from build123d import *

# Parameters (mm, degrees)
EXTRUDE_1_DEPTH        = 20
EXTRUDE_2_DEPTH        = 70
F_1_4_BASE_D           = 3.4
F_1_4_BASE_CBORE_D     = 6.7
F_1_4_BASE_CBORE_DEPTH = 1.65
SKETCH_11_W            = 22
SKETCH_11_H            = 42
CUT_EXTRUDE_1_DEPTH    = 32
CUT_EXTRUDE_2_DEPTH    = 67
SKETCH_15_R            = 5
CUT_EXTRUDE_3_DEPTH    = 70
CUT_EXTRUDE_4_DEPTH    = 2
CUT_EXTRUDE_5_DEPTH    = 3.5


with BuildPart() as part:
    # 草图1 → 凸台-拉伸1 (new body)
    with BuildSketch(Plane(origin=(0, 0, 0), x_dir=(1, 0, 0), z_dir=(0, 1, 0))):
        with BuildLine():
            Line((75.055476805, 35), (35.707142143, 35))
            ThreePointArc((35.707142143, 35), (46.289075964, 18.902948088), (50, 0))
            ThreePointArc((50, 0), (46.289075964, -18.902948088), (35.707142143, -35))
            Line((35.707142143, -35), (75.055476805, -35))
            Line((75.055476805, -35), (75.055476805, 35))
        make_face()
        with BuildLine():
            Line((0.055476805, -35), (0.055476805, 35))
            Line((0.055476805, 35), (35.707142143, 35))
            ThreePointArc((35.707142143, 35), (-50, 0), (35.707142143, -35))
            Line((35.707142143, -35), (0.055476805, -35))
        make_face()
        with BuildLine():
            Line((35.707142143, 35), (0.055476805, 35))
            Line((0.055476805, 35), (0.055476805, -35))
            Line((0.055476805, -35), (35.707142143, -35))
            ThreePointArc((35.707142143, -35), (46.289075964, -18.902948088), (50, 0))
            ThreePointArc((50, 0), (46.289075964, 18.902948088), (35.707142143, 35))
        make_face()
    extrude_1 = extrude(amount=EXTRUDE_1_DEPTH)

    # 草图2 → 凸台-拉伸2 (add)
    with BuildSketch(Plane.XY.offset(35)):
        Polygon((75.055476805, 0), (140.174133177, 114.192122372), (140.174133177, 191.411564081), (120.174133177, 191.411564081), (120.174133177, 109.286292207), (75.055476805, 20), align=None)
    extrude_2 = extrude(amount=-EXTRUDE_2_DEPTH)

    # 镜向1: 凸台-拉伸1, 凸台-拉伸2 across plane
    add(extrude_1.mirror(Plane(origin=(0, 0, 0), x_dir=(0, 0, 1), z_dir=(1, 0, 0))))
    add(extrude_2.mirror(Plane(origin=(0, 0, 0), x_dir=(0, 0, 1), z_dir=(1, 0, 0))))

    # 1/4 六角头螺钉的柱形沉头孔base (through all)
    with Locations(Plane(origin=(0, 20, 0), x_dir=(1, 0, 0), z_dir=(0, 1, 0))):
        with Locations((0, 0)):
            CounterBoreHole(F_1_4_BASE_D / 2, F_1_4_BASE_CBORE_D / 2, F_1_4_BASE_CBORE_DEPTH)

    # 草图11 → 切除-拉伸1 (cut)
    with BuildSketch(Plane(origin=(140.174133177, 0, 0), x_dir=(0, 0, -1), z_dir=(1, 0, 0))):
        with Locations((0, 152.801564081)):
            Rectangle(SKETCH_11_W, SKETCH_11_H)
    extrude(amount=-CUT_EXTRUDE_1_DEPTH, mode=Mode.SUBTRACT)

    # 草图14 → 切除-拉伸2 (cut)
    with BuildSketch(Plane(origin=(140.174133177, 0, 0), x_dir=(0, 0, -1), z_dir=(1, 0, 0))):
        with BuildLine():
            Line((-10, 179.101564081), (10, 179.101564081))
            ThreePointArc((10, 179.101564081), (11, 178.101564081), (10, 177.101564081))
            Line((10, 177.101564081), (-10, 177.101564081))
            ThreePointArc((-10, 177.101564081), (-11, 178.101564081), (-10, 179.101564081))
        make_face()
        with BuildLine():
            Line((-10, 128.501564081), (8.706275956, 128.501564081))
            ThreePointArc((8.706275956, 128.501564081), (9.706275956, 127.501564081), (8.706275956, 126.501564081))
            Line((8.706275956, 126.501564081), (-10, 126.501564081))
            ThreePointArc((-10, 126.501564081), (-11, 127.501564081), (-10, 128.501564081))
        make_face()
    extrude(amount=-CUT_EXTRUDE_2_DEPTH, mode=Mode.SUBTRACT)

    # 草图15 → 切除-拉伸3 (cut)
    with BuildSketch(Plane.ZY.offset(140.174133177)):
        with Locations((0, 172.801564081)):
            Circle(SKETCH_15_R)
    extrude(amount=-CUT_EXTRUDE_3_DEPTH, mode=Mode.SUBTRACT)

    # 草图16 → 切除-拉伸4 (cut)
    with BuildSketch(Plane.XZ):
        with BuildLine():
            Line((-30, 3), (0.784894819, 6.64557965))
            Line((0.784894819, 6.64557965), (31.544487342, 2.792338441))
            ThreePointArc((31.544487342, 2.792338441), (33.403111228, -0.103830779), (31.544487342, -3))
            Line((31.544487342, -3), (0.784894819, -6.64557965))
            Line((0.784894819, -6.64557965), (-30, -3))
            ThreePointArc((-30, -3), (-33, 0), (-30, 3))
        make_face()
    extrude(amount=-CUT_EXTRUDE_4_DEPTH, mode=Mode.SUBTRACT)

    # 草图17 → 切除-拉伸5 (cut)
    with BuildSketch(Plane.XZ):
        Polygon((0.784894819, 6.64557965), (-9.642246975, 5.410786542), (-9.642246975, -5.410786542), (0.784894819, -6.64557965), (11.20346648, -5.410786542), (11.20346648, 5.340449563), align=None)
    extrude(amount=-CUT_EXTRUDE_5_DEPTH, mode=Mode.SUBTRACT)


solid = part.part
For this review, take the finished solid that the model builds, in its own axes (mm). A direction names the side the tool comes from. Round coordinates to 2 decimals unless told otherwise and drop trailing zeros. Write each loop counter-clockwise with the first axis right and the second up, starting at its lowest first coordinate (ties: lowest second). Pieces come first, ordered by that corner, then holes. Notation, with made-up numbers: (24, -27.5) -> (42, -27.5) arc R22 cw to (42, -15.5) -> close; hole circle Ø1 at (58.25, 40). An arc over 180 degrees is marked (long way). Use CSV: the item, a comma, the result in double quotes.
(1) Clearance check with flat-ended pins moving along their axes: P1, Ø4.5, axis at x = 0, z = 0, coming from the +Y side; P2, Ø8, axis at y = 103, z = 20, coming from the +X side; P3, Ø12, axis at x = 111, z = 33.5, coming from the +Y side; P4, Ø1, axis at x = 45, z = -36.5, coming from the +Y side. State where each tip first meets the part, or that it passes through.
Computed values:
P1,"y = 18.35"
P2,"x = 136.07"
P3,"y = 103"
P4,"through"
(2) Consider section A-A, the plane y = 84. Give the boundary of the cut face in (x, z), plus the area to 3 significant figures.
Computed values:
outline,"(-122.96, -35) -> (-107.4, -35) -> (-107.4, 35) -> (-122.96, 35) -> close; (107.4, -35) -> (122.96, -35) -> (122.96, 35) -> (107.4, 35) -> close"
area,"2,180 mm²"
(3) Consider section D-D, the plane x = 27.5. Give the boundary of the cut face in (y, z), plus the area to 3 significant figures.
Computed values:
outline,"(0, -41.76) -> (20, -41.76) -> (20, 41.76) -> (0, 41.76) -> (0, 3.3) -> (2, 3.3) -> (2, -3.48) -> (0, -3.48) -> close"
area,"1,660 mm²"
(4) For faces 5 (the face through (-107, 82, -35)), 6 (the face through (130, 153, 11)), 7 (the face through (-19, 2, 0)), 8 (the face through (-3.347, 19.187, -0.147)), 9 (the face through (1, 20, -12)), list the 3-axis set-ups (+Z, -Z, +X, -X, +Y, -Y) from which the entire face can be reached by the end or side of a thin tool; tool diameter is ignored.
Computed values:
face 5,"-Z, -X, +Y, -Y"
face 6,"+X"
face 7,"-Y"
face 8,"+Y"
face 9,"+Z, -Z, +Y"
(5) To check wall thickness, follow L1, parallel to X at y = 121, z = -23; L2, parallel to Y at x = 72.5, z = -31; L3, parallel to X at y = 29, z = -30. State the ranges of each line that lie inside material, in increasing order. Write a range as [from, to].
Computed values:
L1,"[-140.17, -120.17], [120.17, 140.17]"
L2,"[0, 20]"
L3,"[-91.59, -79.6], [79.6, 91.59]"
(6) Draft analysis for pull direction Z (two halves, no side actions). For faces 1 (the face through (-2, 18.35, -1)), 2 (the face through (0.557, 9.86, -49.997)), 3 (the face through (130, 191.412, 0)), 4 (the face through (130, 126.502, 1)), state which applies: +Z half, -Z half, draft (parallel to the pull), parting line (faces both ways), or undercut.
Computed values:
face 1,"undercut"
face 2,"-Z half"
face 3,"draft"
face 4,"undercut"
(7) Consider section B-B, the plane z = -23.5. Give the boundary of the cut face in (x, y).
Computed values:
outline,"(-140.17, 114.19) -> (-75.06, 0) -> (75.06, 0) -> (140.17, 114.19) -> (140.17, 191.41) -> (120.17, 191.41) -> (120.17, 109.29) -> (75.06, 20) -> (-75.06, 20) -> (-120.17, 109.29) -> (-120.17, 191.41) -> (-140.17, 191.41) -> close"
(8) Consider section C-C, the plane x = -52.5. Give the boundary of the cut face in (y, z).
Computed values:
outline,"(0, -35) -> (20, -35) -> (20, 35) -> (0, 35) -> close"
